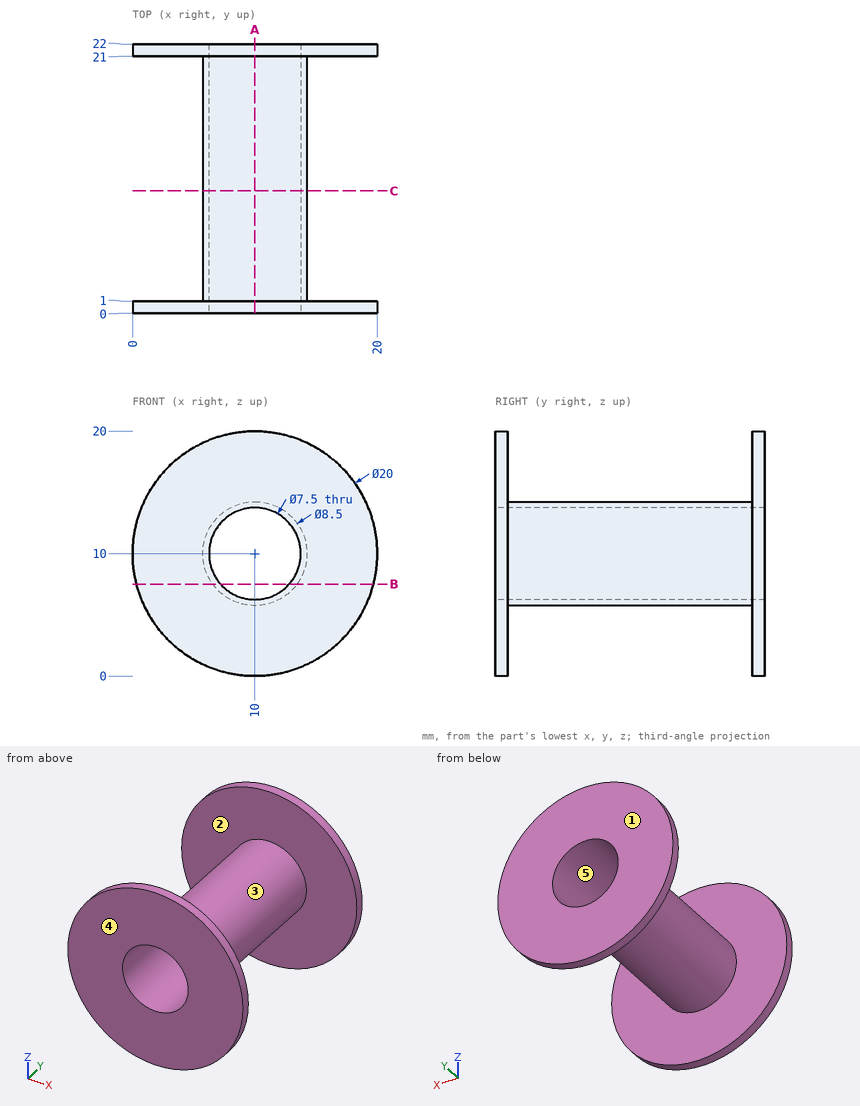
Print and shaded views of the part. All mm, measured from the part's lowest x, y and z. A direction names the side the tool comes from. Give positions to 0.01 mm unless a question says otherwise; leave off trailing zeros. Write each loop counter-clockwise with the first axis right and the second up, starting at its lowest first coordinate (ties: lowest second). Pieces come first, ordered by that corner, then holes. Notation, with made-up numbers: (81, 61.25) -> (101, 61.25) arc R35 cw to (101, 95.25) -> close; hole circle Ø7 at (-31.75, -14.5). An arc over 180 degrees is marked (long way). Write each question's results on one line, items separated by ' | '.
1. Cut at A-A, the plane x = 10. Write the cut outline in (y, z), then the cut area to 3 significant figures.
Geometry check:
outline: (0, 0) -> (1, 0) -> (1, 5.75) -> (21, 5.75) -> (21, 0) -> (22, 0) -> (22, 6.25) -> (0, 6.25) -> close; (0, 13.75) -> (22, 13.75) -> (22, 20) -> (21, 20) -> (21, 14.25) -> (1, 14.25) -> (1, 20) -> (0, 20) -> close | area: 45.0 mm²
2. Wall check: probe 1 along Y at (x, z) = (5.25, 17.5); probe 2 along X at (y, z) = (7.75, 10); probe 3 along Z at (x, y) = (6.75, 7). Give the ranges that are in metal, low to high. Write a range as [from, to].
Geometry check:
probe 1: [0, 1], [21, 22] | probe 2: [5.75, 6.25], [13.75, 14.25] | probe 3: [7.26, 8.13], [11.87, 12.74]
3. Two-plate mould, pull along X, no slides. Class the marked faces 3, 4 and 5: pulls with the +X half, pulls with the -X half, needs draft (parallel to the pull), parting line crosses it, or undercut.
Geometry check:
face 3: parting line crosses it | face 4: needs draft | face 5: undercut
4. Which spindle directions (+Z, -Z, +X, -X, +Y, -Y) get a long thin tool onto all of the face, cutting with end or side? Do the marked faces 1 and 2. Say none if no direction does.
Geometry check:
face 1: +Z, -Z, +X, -X, +Y | face 2: none
5. Cut at B-B, the plane z = 7.5. Write the cut outline in (x, y), then the cut area to 3 significant figures.
Geometry check:
outline: (0.32, 0) -> (7.2, 0) -> (7.2, 22) -> (0.32, 22) -> (0.32, 21) -> (6.56, 21) -> (6.56, 1) -> (0.32, 1) -> close; (12.8, 0) -> (19.68, 0) -> (19.68, 1) -> (13.44, 1) -> (13.44, 21) -> (19.68, 21) -> (19.68, 22) -> (12.8, 22) -> close | area: 53.2 mm²
6. Drop flat-ended pins along their axis: P1, Ø1.5, axis at x = 5.5, y = 4, coming from the +Z side; P2, Ø8, axis at y = 7, z = 7, coming from the +X side; P3, Ø1, axis at y = 15, z = 11, coming from the -X side. Give the stop position or say it passes through.
Geometry check:
P1: z = 12 | P2: x = 14.25 | P3: x = 5.78
7. Cut at C-C, the plane y = 10. Write the cut outline in (x, z).
Geometry check:
outline: circle Ø8.5 at (10, 10); hole circle Ø7.5 at (10, 10)
